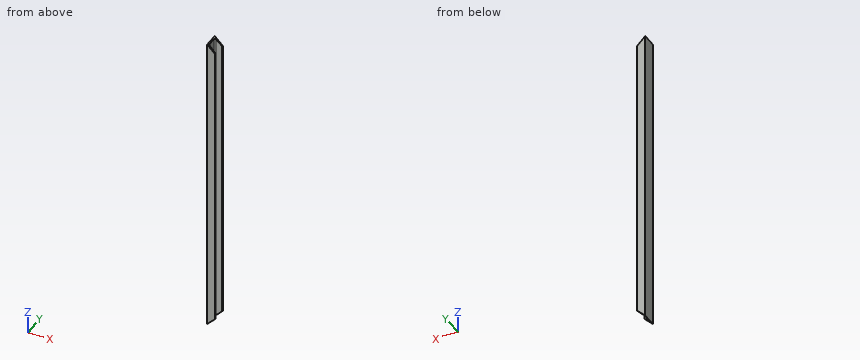
Autodesk Inventor part; units mm, degrees
ref_plane "Начальная плоскость" through (0, 0, -22.5) normal (0, 0, 1) x (1, 0, 0)
ref_plane "Конечная плоскость" through (0, 0, 1682.5) normal (0, 0, 1) x (1, 0, 0)
ref_plane "РабПлоскость4" through (-1.43, 0, -22.5) normal (0.7071, 0, -0.7071) x (-0.7071, 0, -0.7071)
ref_plane "Начальная плоскость" through (0, 0, -22.5) normal (0, 0, 1) x (1, 0, 0)
ref_plane "Конечная плоскость" through (0, 0, 1682.5) normal (0, 0, 1) x (1, 0, 0)
sketch "Эскиз" plane through (0, 0, 0) normal (0, 0, 1) x (1, 0, 0)
  line L0 (-1.43, 0) -> (-1.43, 40)
  line L1 (-1.43, 40) -> (43.57, 40)
  line L2 (43.57, 40) -> (43.57, 38.1774)
  line L3 (39.9881, 34.1993) -> (11.2338, 31.1771)
  line L4 (4.07, 23.221) -> (4.07, 0)
  line L5 (4.07, 0) -> (-1.43, 0) construction
  line L6 (23.82, 40) -> (23.82, 32.5) construction
  line L7 (43.57, 34.5758) -> (43.57, 32.5) construction
  line L8 (43.57, 32.5) -> (23.82, 32.5) construction
  line L9 (0, 15) -> (0, -27) construction
  line L10 (-5.539, 0) -> (16.0067, 0) construction
  line L11 (-1.43, 0) -> (-1.43, -40)
  line L12 (-1.43, -40) -> (43.57, -40)
  line L13 (43.57, -40) -> (43.57, -38.1774)
  line L14 (39.9881, -34.1993) -> (11.2338, -31.1771)
  line L15 (4.07, -23.221) -> (4.07, 0)
  arc A0 (11.2338, 31.1771) -> (4.07, 23.221) centre (12.07, 23.221) ccw
  arc A1 (4.07, -23.221) -> (11.2338, -31.1771) centre (12.07, -23.221) ccw
  arc A2 (39.9881, 34.1993) -> (43.57, 38.1774) centre (39.57, 38.1774) ccw
  arc A3 (43.57, -38.1774) -> (39.9881, -34.1993) centre (39.57, -38.1774) ccw
  line L16 (0, 56) -> (0, -56) construction
  line L17 (-15.5135, 0) -> (54.308, 0) construction
  point P0 (4.07, 30.4242)
  point P1 (43.57, -34.5758)
  point P2 (4.07, -30.4242)
  point P3 (23.82, -40)
  point P4 (23.82, -32.5)
  dimension "d0" = 5.5
  dimension "d1" = 40
  dimension "d2" = 45
  dimension "d3" = 7.5
  dimension "d4" = 19.75
  dimension "d5" = 2.0758
  dimension "d23" = 8
  dimension "d24" = 4
  dimension "d25" = 1.43
extrude "Тело" add sketch "Эскиз" along normal up to surface (1705 mm away) from surface at -22.5
sketch "Sketch3" plane through (0, 0, 0) normal (0, 0, 1) x (1, 0, 0)
  line L0 (0, 0) -> (10, 0)
ref_plane "Work Plane3" through (0, 0, 0) normal (0, -1, 0) x (1, 0, 0)
sketch "Sketch4" plane through (0, 0, 0) normal (0, -1, 0) x (1, 0, 0)
  line L0 (-2, -22.5) -> (12, -22.5)
  line L1 (-2, 1682.5) -> (12, 1682.5)
  dimension "d29" = 1705
ref_plane "РабПлоскость4" through (-1.43, 0, -22.5) normal (0.7071, 0, -0.7071) x (-0.7071, 0, -0.7071)
split "Разделение1" plane through (-1.43, 0, -22.5) removes the side toward (0.7071, 0, -0.7071)
ref_plane "РабПлоскость5" through (-1.43, 0, 1682.5) normal (0.7071, 0, 0.7071) x (0.7071, 0, -0.7071)
split "Разделение2" plane through (-1.43, 0, 1682.5) removes the side toward (0.7071, 0, 0.7071)
equation "\"d0\" = G_T"
equation "\"d1\" = 0.5 * G_H"
equation "\"d2\" = G_W"
equation "\"d3\" = G_T1"
equation "\"d4\" = G_C"
equation "\"d23\" = G_IR"
equation "\"d24\" = G_ER"
equation "\"d25\" = ex"
equation "\"d6\" = G_L"
equation "\"G_W\" = 45"
equation "\"G_T\" = 5.5"
equation "\"G_T1\" = 7.5"
equation "\"G_NG\" = 0.105104"
equation "\"G_ER\" = 4"
equation "\"G_IR\" = 8"
equation "\"G_C\" = 19.75"
equation "\"G_L\" = d29"
equation "\"ex\" = 1.43"
equation "\"G_OFFSET_START\" = 22.5"
equation "\"G_OFFSET_END\" = 22.5"
equation "\"d26\" = -G_OFFSET_START"
equation "\"d27\" = G_OFFSET_END + B_L"
properties part number "ISO 657/11 - CH 80 x 8 - 1705" material "Сталь, мягкая"
Source: CAD feature listing. Evaluate the final solid. Frame: model axes, mm. Give positions to 0.01 mm unless a question says otherwise; leave off trailing zeros. Loops run counter-clockwise (first coordinate to the right, second up) from the corner with the lowest first, then second, coordinate; pieces in that order, holes last. Notation, with made-up numbers: (22.5, 30.25) -> (49.5, 30.25) arc R28 ccw to (49.5, 60.25) -> close; hole circle Ø4 at (0.25, 16). An arc over 180 degrees is marked (long way). Use a Markdown table: item, result. Add a question column.
(1) Section query A-A (x = 31.5). Output: boundary loops of the cut face in (y, z).
(2) Section query B-B (z = 679). Output: boundary loops of the cut face in (x, y), then the cut area to 3 significant figures.
(3) First-contact query: pin 1 Ø10 at (y, z) = (-22.5, 1393) entering from +X; pin 2 Ø2 at (y, z) = (27, 795.5) entering from +X; pin 3 Ø8 at (x, y) = (37.5, 29) entering from -Z. Flat tips, straight axial feed; report the tip coordinate or a pass-through.
(4) Ray query, line 1 (Y direction, x = 11.5, z = 337.5); line 2 (Y direction, x = 37.5, z = 1348.5); line 3 (X direction, y = 17.5, z = 867.5). Return the intervals inside material, ascending.
(5) Section query C-C (y = 1). Output: boundary loops of the cut face in (x, z), then the cut area to 3 significant figures.
Checked values:
| question | item | result |
|---|---|---|
| 1 | outline | (-40, 10.43) -> (-33.31, 10.43) -> (-33.31, 1649.57) -> (-40, 1649.57) -> close; (33.31, 10.43) -> (40, 10.43) -> (40, 1649.57) -> (33.31, 1649.57) -> close |
| 2 | outline | (-1.43, -40) -> (43.57, -40) -> (43.57, -38.18) arc R4 ccw to (39.99, -34.2) -> (11.23, -31.18) arc R8 cw to (4.07, -23.22) -> (4.07, 23.22) arc R8 cw to (11.23, 31.18) -> (39.99, 34.2) arc R4 ccw to (43.57, 38.18) -> (43.57, 40) -> (-1.43, 40) -> close |
| 2 | area | 1,050 mm^2 |
| 3 | pin 1 | x = 5.31 |
| 3 | pin 2 | x = 5.65 |
| 3 | pin 3 | through |
| 4 | line 1 | -40 to -31.21, 31.21 to 40 |
| 4 | line 2 | -40 to -33.94, 33.94 to 40 |
| 4 | line 3 | -1.43 to 4.07 |
| 5 | outline | (-1.43, -22.5) -> (4.07, -17) -> (4.07, 1677) -> (-1.43, 1682.5) -> close |
| 5 | area | 9,350 mm^2 |
